```python
from build123d import *

# Parameters (mm, degrees)
SKETCH3_R           = 2.5
BOSS_EXTRUDE1_DEPTH = 10


with BuildPart() as part:
    # Sketch3 → Boss-Extrude1 (new body)
    with BuildSketch(Plane.XY):
        with BuildLine():
            Line((0, 5), (50, 5))
            ThreePointArc((50, 5), (55, 0), (50, -5))
            Line((50, -5), (2.071067812, -5))
            Line((2.071067812, -5), (-58.388347648, -65.45941546))
            ThreePointArc((-58.388347648, -65.45941546), (-62.723802675, -71.947882437), (-64.246212025, -79.601551084))
            Line((-64.246212025, -79.601551084), (-64.246212025, -167.175144213))
            ThreePointArc((-64.246212025, -167.175144213), (-69.246212025, -172.175144213), (-74.246212025, -167.175144213))
            Line((-74.246212025, -167.175144213), (-74.246212025, -75.45941546))
            ThreePointArc((-74.246212025, -75.45941546), (-72.723802675, -67.805746813), (-68.388347648, -61.317279836))
            Line((-68.388347648, -61.317279836), (-3.535533906, 3.535533906))
            ThreePointArc((-3.535533906, 3.535533906), (-1.913417162, 4.619397663), (0, 5))
        make_face()
        Circle(SKETCH3_R, mode=Mode.SUBTRACT)
        with Locations((50, 0)):
            Circle(SKETCH3_R, mode=Mode.SUBTRACT)
    extrude(amount=BOSS_EXTRUDE1_DEPTH)


solid = part.part
```
Can you work these out from the model? Positions are in its coordinate system, mm. A direction names the side the tool comes from. Round coordinates to 2 decimals unless told otherwise and drop trailing zeros. Loops run counter-clockwise (first coordinate to the right, second up) from the corner with the lowest first, then second, coordinate; pieces in that order, holes last. Notation, with made-up numbers: (67, -21) -> (102, -21) arc R17 cw to (102, -7) -> close; hole circle Ø2 at (-28.5, 59). An arc over 180 degrees is marked (long way). Answer in a Markdown table with one row per item.
Item 1: If I drill on probe 1 along Y at (x, z) = (50, 2); probe 2 along Y at (x, z) = (30, 2.5); probe 3 along X at (y, z) = (-89, 5), over which ranges is the centre line in solid material (lowest first)?
Answer block:
| item | result |
|---|---|
| probe 1 | -5 to -2.5, 2.5 to 5 |
| probe 2 | -5 to 5 |
| probe 3 | -74.25 to -64.25 |
Item 2: On a 3-axis mill with a long thin cutter (end or side, diameter ignored), from which of +Z, -Z, +X, -X, +Y, -Y can I reach the whole of each face in a straight line? I mean faces 5 (the cylindrical face through (-1.94, 4.61, 4.93)), 6 (the flat face through (-64.246, -123, 5)). Say none if no direction works.
Answer block:
| item | result |
|---|---|
| face 5 | +Z, -Z, -X, +Y |
| face 6 | +Z, -Z, +X, -Y |
Item 3: Suppose I cut it at A-A, the plane z = 6. List the corners of the cut face in (x, y) for me.
Answer block:
| item | result |
|---|---|
| outline | (-74.25, -167.18) arc R5 ccw to (-64.25, -167.18) -> (-64.25, -79.6) arc R20 cw to (-58.39, -65.46) -> (2.07, -5) -> (50, -5) arc R5 ccw to (50, 5) -> (0, 5) arc R5 ccw to (-3.54, 3.54) -> (-68.39, -61.32) arc R20 ccw to (-74.25, -75.46) -> close; hole circle Ø5 at (0, 0); hole circle Ø5 at (50, 0) |
Item 4: Suppose I cut it at D-D, the plane x = -9. List the corners of the cut face in (y, z) for me.
Answer block:
| item | result |
|---|---|
| outline | (-16.07, 0) -> (-1.93, 0) -> (-1.93, 10) -> (-16.07, 10) -> close |
Item 5: Suppose I cut it at B-B, the plane y = 0. List the corners of the cut face in (x, z) for me, plus the area to 3 significant figures.
Answer block:
| item | result |
|---|---|
| outline | (-7.07, 0) -> (-2.5, 0) -> (-2.5, 10) -> (-7.07, 10) -> close; (2.5, 0) -> (47.5, 0) -> (47.5, 10) -> (2.5, 10) -> close; (52.5, 0) -> (55, 0) -> (55, 10) -> (52.5, 10) -> close |
| area | 521 mm² |
Item 6: Will these pins go through, and if not, where does the flat tip stop? P1, Ø6, axis at x = -31.5, z = 4.5, coming from the -Y side; P2, Ø4, axis at y = -106, z = 6, coming from the +X side; P3, Ø4, axis at y = -19, z = 2, coming from the -X side.
Answer block:
| item | result |
|---|---|
| P1 | y = -41.57 |
| P2 | x = -64.25 |
| P3 | x = -28.07 |
Item 7: Suppose I cut it at C-C, the plane y = -126.5. List the corners of the cut face in (x, z) for me, plus the area to 3 significant figures.
Answer block:
| item | result |
|---|---|
| outline | (-74.25, 0) -> (-64.25, 0) -> (-64.25, 10) -> (-74.25, 10) -> close |
| area | 100 mm² |
Item 8: We'd pull the mould along X, two halves only. Please class faces 1 (the cylindrical face through (52.31, -0.96, 4.93)), 2 (the cylindrical face through (-0.54, -2.44, 4.93)), 3 (the flat face through (25, 5, 5)), 4 (the cylindrical face through (55, 0, 5)): released by +X, released by -X, zero draft, split by the parting line, or undercut.
Answer block:
| item | result |
|---|---|
| face 1 | undercut |
| face 2 | undercut |
| face 3 | zero draft |
| face 4 | released by +X |
